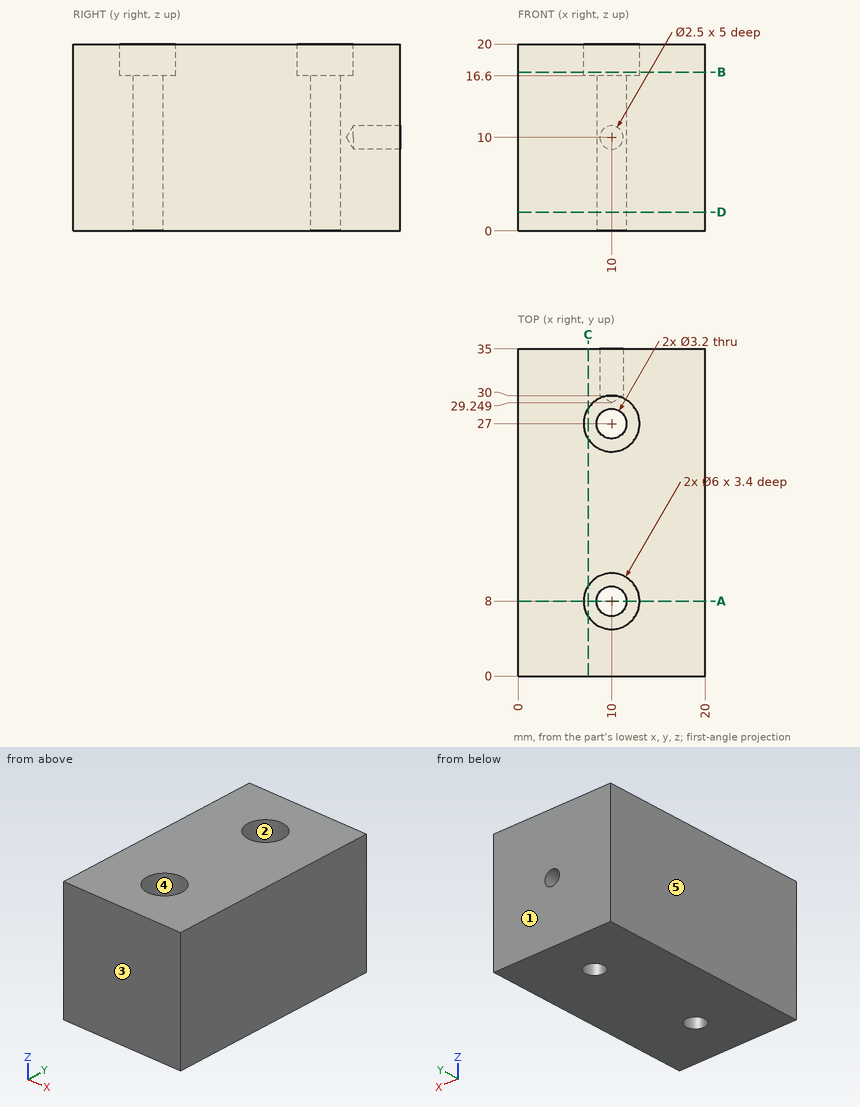
Design review of the part shown in the three views and the two pictorial views. Dimensions are in mm from the part's minimum x, y and z. A direction names the side the tool comes from. Round coordinates to 2 decimals unless told otherwise and drop trailing zeros. Loops run counter-clockwise (first coordinate to the right, second up) from the corner with the lowest first, then second, coordinate; pieces in that order, holes last.
Q1. Add section D-D on z = 2. Write out the cut boundary in (x, y), plus the area to 3 significant figures.
Result sheet:
outline: (0, 0) - (20, 0) - (20, 35) - (0, 35) - close; hole circle Ø3.2 at (10, 8); hole circle Ø3.2 at (10, 27)
area: 684 mm2
Q2. Machinability: for the marked faces 1 and 2, which of the approach directions +Z, -Z, +X, -X, +Y, -Y give a long, thin tool a straight path to every point of the face, cutting with its end or side? Answer none if there is none.
Result sheet:
face 1: +Z, -Z, +X, -X, +Y
face 2: +Z
Q3. Mouldability with a two-part tool opening along X and no side actions: class the marked faces 3, 4 and 5 as +X half, -X half, draft (parallel to the pull), parting line (faces both ways), or undercut.
Result sheet:
face 3: draft
face 4: undercut
face 5: -X half
Q4. To check wall thickness, follow line 1 along Y through (x, z) = (10, 18.7); line 2 along Y through (x, z) = (10, 8.25); line 3 along Z through (x, y) = (10, 32.1). State the ranges of each line that lie inside material, in increasing order.
Result sheet:
line 1: y = 0 to 5, 11 to 24, 30 to 35
line 2: y = 0 to 6.4, 9.6 to 25.4, 28.6 to 35
line 3: z = 0 to 8.75, 11.25 to 20
Q5. Add section C-C on x = 7.5. Write out the cut boundary in (y, z).
Result sheet:
outline: (0, 0) - (35, 0) - (35, 20) - (28.66, 20) - (28.66, 16.6) - (25.34, 16.6) - (25.34, 20) - (9.66, 20) - (9.66, 16.6) - (6.34, 16.6) - (6.34, 20) - (0, 20) - close
Q6. Add section A-A on y = 8. Write out the cut boundary in (x, z).
Result sheet:
outline: (0, 0) - (8.4, 0) - (8.4, 16.6) - (7, 16.6) - (7, 20) - (0, 20) - close; (11.6, 0) - (20, 0) - (20, 20) - (13, 20) - (13, 16.6) - (11.6, 16.6) - close
Q7. Insertion check: pin 1 Ø3 at (x, z) = (10, 10) entering from +Y. The pin has a flat end and moves straight along its axis. Give the tip position at first contact, or say it passes through.
Result sheet:
pin 1: stops at y = 35
Q8. Add section B-B on z = 17. Write out the cut boundary in (x, y), plus the area to 3 significant figures.
Result sheet:
outline: (0, 0) - (20, 0) - (20, 35) - (0, 35) - close; hole circle Ø6 at (10, 8); hole circle Ø6 at (10, 27)
area: 643 mm2
